CAD build for the part. Positions are in the model's coordinates, mm. A direction names the side the tool comes from. Round coordinates to 2 decimals unless told otherwise and drop trailing zeros. Loops run counter-clockwise (first coordinate to the right, second up) from the corner with the lowest first, then second, coordinate; pieces in that order, holes last.
```python
from build123d import *

# Parameters (mm, degrees)
BOSS_EXTRU_1_DEPTH           = 1.6
ESQUISSE3_W                  = 3.45
ESQUISSE3_H                  = 3.45
BOSS_EXTRU_2_DEPTH           = 3
ESQUISSE4_W                  = 3.45
ESQUISSE4_H                  = 3.45
BOSS_EXTRU_3_DEPTH           = 3
ESQUISSE5_W                  = 3
ESQUISSE5_H                  = 3
BOSS_EXTRU_4_DEPTH           = 3
ESQUISSE6_W                  = 1.72
ESQUISSE6_H                  = 2.12
BOSS_EXTRU_5_DEPTH           = 1
ENL_V_MAT_EXTRU_1_DEPTH      = 95.387499172
ENL_V_MAT_EXTRU_1_DEPTH_BACK = 95.387499172
ESQUISSE7_R                  = 2.25
ESQUISSE7_R_2                = 1.65
ESQUISSE8_W                  = 25
ESQUISSE8_H                  = 25
BOSS_EXTRU_6_DEPTH           = 11.5
ESQUISSE9_W                  = 10
ESQUISSE9_H                  = 10
BOSS_EXTRU_7_DEPTH           = 5
ESQUISSE10_W                 = 9.65005
ESQUISSE10_H                 = 4.37005
ESQUISSE10_W_2               = 9.65
BOSS_EXTRU_8_DEPTH           = 5


with BuildPart() as part:
    # Esquisse2 → Boss.-Extru.1 (new body)
    with BuildSketch(Plane.XY):
        with BuildLine():
            Line((0, 3), (0, 47))
            ThreePointArc((0, 47), (0.878679656, 49.121320344), (3, 50))
            Line((3, 50), (77, 50))
            ThreePointArc((77, 50), (79.121320344, 49.121320344), (80, 47))
            Line((80, 47), (80, 3))
            ThreePointArc((80, 3), (79.121320344, 0.878679656), (77, 0))
            Line((77, 0), (59.2426, 0))
            ThreePointArc((59.2426, 0), (58.094558305, -0.228374693), (57.1213, -0.8787))
            Line((57.1213, -0.8787), (48.8787, -9.1213))
            ThreePointArc((48.8787, -9.1213), (47.905441695, -9.771625307), (46.7574, -10))
            Line((46.7574, -10), (29.2426, -10))
            ThreePointArc((29.2426, -10), (28.094558305, -9.771625307), (27.1213, -9.1213))
            Line((27.1213, -9.1213), (18.8787, -0.8787))
            ThreePointArc((18.8787, -0.8787), (17.905441695, -0.228374693), (16.7574, 0))
            Line((16.7574, 0), (3, 0))
            ThreePointArc((3, 0), (0.878679656, 0.878679656), (0, 3))
        make_face()
    extrude(amount=-BOSS_EXTRU_1_DEPTH)

    # Esquisse3 → Boss.-Extru.2 (add)
    with BuildSketch(Plane.XY):
        with Locations((10, 10)):
            Rectangle(ESQUISSE3_W, ESQUISSE3_H)
        with Locations((10, 30)):
            Rectangle(ESQUISSE3_W, ESQUISSE3_H)
    extrude(amount=BOSS_EXTRU_2_DEPTH)

    # Esquisse4 → Boss.-Extru.3 (add)
    with BuildSketch(Plane.XY):
        with Locations((70, 10)):
            Rectangle(ESQUISSE4_W, ESQUISSE4_H)
        with Locations((70, 30)):
            Rectangle(ESQUISSE4_W, ESQUISSE4_H)
    extrude(amount=BOSS_EXTRU_3_DEPTH)

    # Esquisse5 → Boss.-Extru.4 (add)
    with BuildSketch(Plane.XY):
        with Locations((40, 25.5)):
            Rectangle(ESQUISSE5_W, ESQUISSE5_H)
    extrude(amount=BOSS_EXTRU_4_DEPTH)

    # Esquisse6 → Boss.-Extru.5 (add)
    with BuildSketch(Plane.XY):
        with Locations((40, 13.75)):
            Rectangle(ESQUISSE6_W, ESQUISSE6_H)
    extrude(amount=BOSS_EXTRU_5_DEPTH)

    # Esquisse7 → Enlèv. mat.-Extru.1 (cut, two sides: drawn at the far end of the back side and taken through both)
    with BuildSketch(Plane.XY.offset(-ENL_V_MAT_EXTRU_1_DEPTH_BACK)):
        with Locations((20, 20)):
            Circle(ESQUISSE7_R)
        with Locations((60, 20)):
            Circle(ESQUISSE7_R)
        with Locations((33, 29)):
            Circle(ESQUISSE7_R_2)
        with Locations((52, 10)):
            Circle(ESQUISSE7_R_2)
    extrude(amount=ENL_V_MAT_EXTRU_1_DEPTH + ENL_V_MAT_EXTRU_1_DEPTH_BACK, mode=Mode.SUBTRACT)

    # Esquisse8 → Boss.-Extru.6 (add)
    with BuildSketch(Plane(origin=(0, 0, -1.6), x_dir=(-1, 0, 0), z_dir=(0, 0, -1))):
        with Locations((-42.5, 19.5)):
            Rectangle(ESQUISSE8_W, ESQUISSE8_H)
    extrude(amount=BOSS_EXTRU_6_DEPTH)

    # Esquisse9 → Boss.-Extru.7 (add)
    with BuildSketch(Plane(origin=(0, 0, -1.6), x_dir=(-1, 0, 0), z_dir=(0, 0, -1))):
        with Locations((-16.5, 43)):
            Rectangle(ESQUISSE9_W, ESQUISSE9_H)
        with Locations((-35, 42.75)):
            Rectangle(ESQUISSE9_W, ESQUISSE9_H)
        with Locations((-54.45, 42.72)):
            Rectangle(ESQUISSE9_W, ESQUISSE9_H)
        with Locations((-73.5, 42.75)):
            Rectangle(ESQUISSE9_W, ESQUISSE9_H)
    extrude(amount=BOSS_EXTRU_7_DEPTH)

    # Esquisse10 → Boss.-Extru.8 (add)
    with BuildSketch(Plane(origin=(0, 0, -1.6), x_dir=(-1, 0, 0), z_dir=(0, 0, -1))):
        with Locations((-31.500025, -3.715025)):
            Rectangle(ESQUISSE10_W, ESQUISSE10_H)
        with Locations((-44.75, -3.715025)):
            Rectangle(ESQUISSE10_W_2, ESQUISSE10_H)
    extrude(amount=BOSS_EXTRU_8_DEPTH)


solid = part.part
```
Item 1: Cut at C-C, the plane z = -3.75. Give the cut face in (x, y) (3 decimals), plus the area to 3 significant figures.
Answers follow:
outline: (11.5, 38) - (21.5, 38) - (21.5, 48) - (11.5, 48) - close; (26.675, -5.9) - (36.325, -5.9) - (36.325, -1.53) - (26.675, -1.53) - close; (30, 7) - (55, 7) - (55, 32) - (30, 32) - close; (30, 37.75) - (40, 37.75) - (40, 47.75) - (30, 47.75) - close; (39.925, -5.9) - (49.575, -5.9) - (49.575, -1.53) - (39.925, -1.53) - close; (49.45, 37.72) - (59.45, 37.72) - (59.45, 47.72) - (49.45, 47.72) - close; (68.5, 37.75) - (78.5, 37.75) - (78.5, 47.75) - (68.5, 47.75) - close
area: 1,110 mm2
Item 2: Cut at B-B, the plane y = 20. Give the cut face in (x, z), plus the area to 3 significant figures.
Answers follow:
outline: (0, -1.6) - (17.75, -1.6) - (17.75, 0) - (0, 0) - close; (22.25, -1.6) - (30, -1.6) - (30, -13.1) - (55, -13.1) - (55, -1.6) - (57.75, -1.6) - (57.75, 0) - (22.25, 0) - close; (62.25, -1.6) - (80, -1.6) - (80, 0) - (62.25, 0) - close
area: 401 mm2
Item 3: Cut at A-A, the plane x = 20. Give the cut face in (y, z), plus the area to 3 significant figures.
Answers follow:
outline: (-2, -1.6) - (17.75, -1.6) - (17.75, 0) - (-2, 0) - close; (22.25, -1.6) - (38, -1.6) - (38, -6.6) - (48, -6.6) - (48, -1.6) - (50, -1.6) - (50, 0) - (22.25, 0) - close
area: 126 mm2
Item 4: Flat gauge pins, fed straight in: P1, Ø0.9, axis at x = 40, y = 13.5, coming from the +Z side; P2, Ø1.5, axis at y = 41, z = -5, coming from the -X side; P3, Ø3, axis at x = 71, z = -3, coming from the -Y side. Where does each tip first touch, or does it go through?
Answers follow:
P1: stops at z = 1
P2: stops at x = 11.5
P3: stops at y = 0
Item 5: Two-plate mould, pull along Y, no slides. Class faces 5 (the cylindrical face through (58.214, 18.631, -0.811)), 6 (the cylindrical face through (0.9, 0.86, -0.79)), 7 (the flat face through (8.275, 10, 1)), 8 (the cylindrical face through (32.785, 30.636, -0.811)): released by +Y, released by -Y, zero draft, split by the parting line, or undercut.
Answers follow:
face 5: undercut
face 6: released by -Y
face 7: zero draft
face 8: undercut
Item 6: 3-axis set-ups, long thin cutter, end or side, ignore diameter. For faces 1 (the flat face through (68.5, 43, -4)), 2 (the flat face through (17, 48, -4)), 3 (the flat face through (11.725, 10, 1)), 4 (the flat face through (10, 0, -1)): which of +Z, -Z, +X, -X, +Y, -Y reach the whole face in a straight line?
Answers follow:
face 1: -Z, +Y, -Y
face 2: -Z, +X, -X, +Y
face 3: +Z, +Y, -Y
face 4: +Z, -Z, -X, -Y
Item 7: Probe line 1 (X direction, y = 20, z = -0.6); line 2 (X direction, y = 29, z = -0.4); line 3 (Y direction, x = 60, z = -0.7). List the from-to ranges inside material, lowest first.
Answers follow:
line 1: x = 0 to 17.75, 22.25 to 57.75, 62.25 to 80
line 2: x = 0 to 31.35, 34.65 to 80
line 3: y = 0 to 17.75, 22.25 to 50
Item 8: Cut at D-D, the plane x = 74. Give the cut face in (y, z).
Answers follow:
outline: (0, -1.6) - (37.75, -1.6) - (37.75, -6.6) - (47.75, -6.6) - (47.75, -1.6) - (50, -1.6) - (50, 0) - (0, 0) - close
